from build123d import *

# Parameters (mm, degrees)
CUT_EXTRUDE2_DEPTH      = 165.71500296
CUT_EXTRUDE2_DEPTH_BACK = 165.71500296
SKETCH3_W               = 77.6
SKETCH3_H               = 9.49


with BuildPart() as part:
    # Sketch1 → Revolve1 (revolve)
    with BuildSketch(Plane.XY, mode=Mode.PRIVATE) as revolve1_sk:
        Polygon((161.48, 0), (161.48, 18.68), (43.78, 18.68), (43.78, 22.97), (30, 22.97), (30, 18.68), (0, 18.68), (0, 0), align=None)
    revolve(revolve1_sk.sketch.rotate(Axis((0, 0, 0), (1, 0, 0)), 180), axis=Axis((0, 0, 0), (1, 0, 0)))

    # Sketch3 → Cut-Extrude2 (cut, two sides: drawn at the far end of the back side and taken through both)
    with BuildSketch(Plane(origin=(0, 0, 0), x_dir=(1, 0, 0), z_dir=(0, 1, 0)).offset(-CUT_EXTRUDE2_DEPTH_BACK)):
        with Locations((114.69, 0)):
            Rectangle(SKETCH3_W, SKETCH3_H)
    extrude(amount=CUT_EXTRUDE2_DEPTH + CUT_EXTRUDE2_DEPTH_BACK, mode=Mode.SUBTRACT)


solid = part.part
For this review, take the finished solid that the model builds, in its own axes (mm). A direction names the side the tool comes from. Round coordinates to 2 decimals unless told otherwise and drop trailing zeros. Order: outer loops, then holes, each group sorted by start corner. A loop starts at its lowest first (then second) coordinate and runs counter-clockwise, first axis right, second up. Notation, with made-up numbers: M 43.25,-35 L 89.25,-35 A6 ccw 89.25,-24 Z; hole C -17,-2.5 d1. An arc over 180 degrees is marked long. Write each question's results on one line, items separated by ' | '. Start each with the question number.
1. Add section B-B (y = -14.5). State the section outline as (x, z) points (3 decimals).
2. Draft analysis for pull direction Z (two halves, no side actions). For faces 1 (the face through (36.79, -10.6, 20.38)), 2 (the face through (0, 0, 0)), 3 (the face through (114, 0, -4.745)), state which applies: pulls with the +Z half, pulls with the -Z half, needs draft (parallel to the pull), parting line crosses it, or undercut.
3. Tool access review of faces 4 (the face through (101.806, -17.817, -5.611)), 5 (the face through (30, -3, 19)), 6 (the face through (75.89, 0, 0)), 7 (the face through (161.48, 0, 0)): name each direction out of +Z, -Z, +X, -X, +Y, -Y from which nothing blocks a thin tool from reaching the whole face with its end or side.
4. Add section D-D (z = 11.5). State the section outline as (x, y) points.
5. To check wall thickness, follow L1, parallel to X at y = -15.5, z = 1.5; L2, parallel to X at y = 1, z = -20; L3, parallel to Z at x = 146, y = 16.5 (3 decimals). State the ranges of each line that lie inside material, in increasing order. Write a range as [from, to].
6. Add section A-A (z = 0). State the section outline as (x, y) points.
7. Clearance check with flat-ended pins moving along their axes: pin 1 Ø4 at (y, z) = (-15.5, 14) entering from +X; pin 2 Ø5 at (x, z) = (75.5, 12.5) entering from -Y; pin 3 Ø5 at (x, z) = (18.5, 15) entering from -Y; pin 4 Ø8 at (y, z) = (5, -4) entering from -X. State where each tip first meets the part, or that it passes through.
8. Add section C-C (x = 57). State the section outline as (y, z) points, then the cut area to 3 significant figures.
Output values:
1) outline: M 0,-11.777 L 30,-11.777 L 30,-17.815 L 43.78,-17.815 L 43.78,-11.777 L 161.48,-11.777 L 161.48,11.777 L 43.78,11.777 L 43.78,17.815 L 30,17.815 L 30,11.777 L 0,11.777 Z; hole M 75.89,-4.745 L 153.49,-4.745 L 153.49,4.745 L 75.89,4.745 Z
2) face 1: parting line crosses it | face 2: needs draft | face 3: undercut
3) face 4: +X | face 5: -X | face 6: +Y, -Y | face 7: +Z, -Z, +X, +Y, -Y
4) outline: M 0,-14.72 L 30,-14.72 L 30,-19.88 L 43.78,-19.88 L 43.78,-14.72 L 161.48,-14.72 L 161.48,14.72 L 43.78,14.72 L 43.78,19.88 L 30,19.88 L 30,14.72 L 0,14.72 Z
5) L1: [0, 75.89], [153.49, 161.48] | L2: [30, 43.78] | L3: [-8.757, -4.745], [4.745, 8.757]
6) outline: M 0,-18.68 L 30,-18.68 L 30,-22.97 L 43.78,-22.97 L 43.78,-18.68 L 75.89,-18.68 L 75.89,18.68 L 43.78,18.68 L 43.78,22.97 L 30,22.97 L 30,18.68 L 0,18.68 Z; M 153.49,-18.68 L 161.48,-18.68 L 161.48,18.68 L 153.49,18.68 Z
7) pin 1: x = 43.78 | pin 2: y = -15.78 | pin 3: y = -13.88 | pin 4: x = 0
8) outline: C 0,0 d37.36 | area: 1,100 mm^2
